CAD build for the part. Positions are in the model's coordinates, mm. Face numbers are marked on the shaded views. A direction names the side the tool comes from. Give positions to 0.01 mm unless a question says otherwise; leave off trailing zeros. Order: outer loops, then holes, each group sorted by start corner. A loop starts at its lowest first (then second) coordinate and runs counter-clockwise, first axis right, second up. Notation, with made-up numbers: (28.25, 21) -> (35.25, 21) arc R13 ccw to (35.25, 36) -> close; hole circle Ø3 at (-11, 14.5). An arc over 180 degrees is marked (long way). Use one line per item in the form item = value. Start each with the question number.
1) Drop flat-ended pins along their axis: P1, Ø4, axis at x = 6, z = 3.5, coming from the -Y side; P2, Ø5.5, axis at x = -1.5, y = -8.5, coming from the +Z side; P3, Ø5.5, axis at x = -12, z = 4, coming from the -Y side; P4, Ø3.5, axis at x = -0.5, z = 5.5, coming from the +Y side. Give the stop position or say it passes through.
2) Probe line 1 (Y direction, x = -10, z = 9); line 2 (X direction, y = -7, z = 6); line 3 (X direction, y = -5.75, z = 2). List the from-to ranges inside material, lowest first.
3) Cut at D-D, the plane x = -20. Give the cut face in (y, z).
4) Cut at A-A, the plane y = -13.25. Give the cut face in (x, z), and give its area (3 significant figures).
5) Mould opens along Y. For the marked faces 4, 5, 6 and 7 say: pulls with the +Y half, pulls with the -Y half, needs draft (parallel to the pull), parting line crosses it, or undercut.
6) Cut at B-B, the plane z = 8. Give the cut face in (x, y), and give its area (3 significant figures).
7) Cut at C-C, the plane x = 0. Give the cut face in (y, z).
8) Tool access for the marked faces 1, 2 and 3: list every direction of +Z, -Z, +X, -X, +Y, -Y with a clear straight run to the whole face (end or side of a thin tool).
from build123d import *
from build123d.topology import SkipClean

# Parameters (mm, degrees)
SKETCH1_R           = 7
BOSS_EXTRUDE1_DEPTH = 13
SKETCH2_R           = 7
BOSS_EXTRUDE2_DEPTH = 3
SKETCH3_R           = 3
CUT_EXTRUDE1_DEPTH  = 13


with BuildPart() as part:
    # Sketch1 → Boss-Extrude1 (new body)
    with BuildSketch(Plane.XY):
        with BuildLine():
            ThreePointArc((16.808917195, -9.124391157), (14.337583538, -12.994121317), (10, -14.5))
            Line((10, -14.5), (15, -14.5))
            Line((15, -14.5), (15, -17.75))
            Line((15, -17.75), (30, -17.75))
            Line((30, -17.75), (30, -14.75))
            Line((30, -14.75), (16.808917195, -9.124391157))
        make_face()
        with Locations((10, -7.5)):
            Circle(SKETCH1_R)
        with BuildLine():
            Line((0, -10), (3.461651585, -10))
            ThreePointArc((3.461651585, -10), (3, -7.5), (3.461651585, -5))
            Line((3.461651585, -5), (0, -5))
            Line((0, -5), (0, -10))
        make_face()
    extrude(amount=BOSS_EXTRUDE1_DEPTH)

    # Sketch2 → Boss-Extrude2 (add)
    with BuildSketch(Plane.XY.offset(13)):
        with Locations(Location((10, -7.5, 0), (0, 0, 200.924832428))):
            Circle(SKETCH2_R)
    extrude(amount=BOSS_EXTRUDE2_DEPTH)

    # Sketch3 → Cut-Extrude1 (cut)
    with BuildSketch(Plane.XY):
        with Locations((10, -7.5)):
            Circle(SKETCH3_R)
        with BuildLine():
            Line((16.808917195, -9.124391157), (17.20120329, -8.204547899))
            Line((17.20120329, -8.204547899), (12.752773317, -6.307423351))
            ThreePointArc((12.752773317, -6.307423351), (12.937543187, -6.891033643), (13, -7.5))
            Line((13, -7.5), (16.808917195, -9.124391157))
        make_face()
    extrude(amount=CUT_EXTRUDE1_DEPTH, mode=Mode.SUBTRACT)

    # Mirror1: part across plane


with BuildPart() as part_1:
    with SkipClean():  # the faces are left unmerged after this step: merging them gives an invalid solid
        add(part.part)
        add(part.part.mirror(Plane(origin=(0, 0, 0), x_dir=(0, 0, 1), z_dir=(1, 0, 0))))


solid = part_1.part
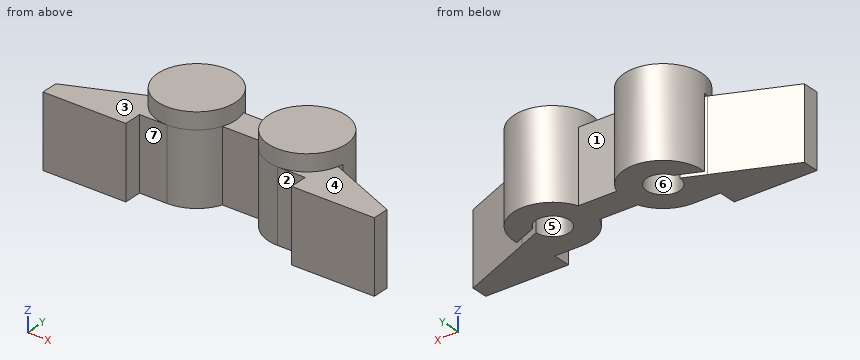
Result:
q1.P1 = -14.21
q1.P2 = 16
q1.P3 = -14.5
q1.P4 = -5
q2.line_1 = -14.5 to -10.5, -4.5 to -0.5
q2.line_2 = -16.98 to -14.38, -7.04 to 7.04, 14.38 to 16.98
q2.line_3 = -16.78 to -12.44, -7.56 to 7.56, 12.44 to 16.78
q3.outline = (-17.75, 0) -> (-10.49, 0) -> (-10.49, 13) -> (-17.75, 13) -> close
q4.outline = (-26.48, 0) -> (-6.01, 0) -> (-6.01, 16) -> (-13.99, 16) -> (-13.99, 13) -> (-26.48, 13) -> close; (6.01, 0) -> (26.48, 0) -> (26.48, 13) -> (13.99, 13) -> (13.99, 16) -> (6.01, 16) -> close
q4.area = 580 mm²
q5.face_4 = needs draft
q5.face_5 = undercut
q5.face_6 = undercut
q5.face_7 = pulls with the -Y half
q6.outline = (-30, -17.75) -> (-15, -17.75) -> (-15, -14.5) -> (-10, -14.5) arc R7 ccw to (-3.46, -10) -> (3.46, -10) arc R7 ccw to (10, -14.5) -> (15, -14.5) -> (15, -17.75) -> (30, -17.75) -> (30, -14.75) -> (13, -7.5) arc R3 cw (long way) to (12.75, -6.31) -> (16.97, -8.11) arc R7 ccw to (3.46, -5) -> (-3.46, -5) arc R7 ccw to (-16.97, -8.11) -> (-12.75, -6.31) arc R3 cw (long way) to (-13, -7.5) -> (-30, -14.75) -> close
q6.area = 458 mm²
q7.outline = (-10, 0) -> (-5, 0) -> (-5, 13) -> (-10, 13) -> close
q8.face_1 = +Z, -Z, +Y
q8.face_2 = +Z, -Z, -Y
q8.face_3 = +Z, -X, -Y
